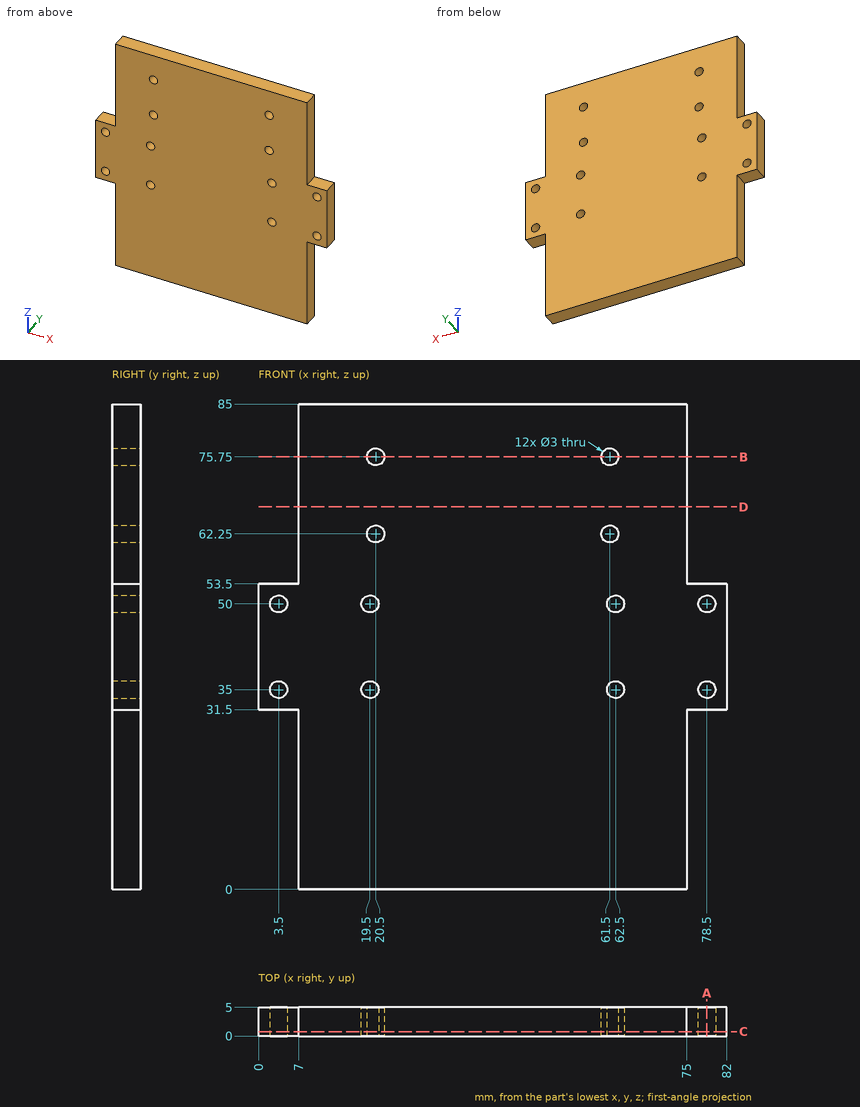
Print and shaded views of the part. All mm, measured from the part's lowest x, y and z. Round coordinates to 2 decimals unless told otherwise and drop trailing zeros. Order: outer loops, then holes, each group sorted by start corner. A loop starts at its lowest first (then second) coordinate and runs counter-clockwise, first axis right, second up.
Q1. Slice it at D-D (z = 67). Write the cut outline in (x, y), and give its area (3 significant figures).
Q2. Slice it at A-A (x = 78.5). Write the cut outline in (y, z), and give its area (3 significant figures).
Q3. Wall check: L1, parallel to X at y = 1.15, z = 76; L2, parallel to Z at x = 3, y = 2.9; L3, parallel to Z at x = 20.5, y = 1.7. Give the ranges that are in metal, low to high.
Q4. Drop flat-ended pins along their axis: pin 1 (5 mm diameter, centred on x = 62.5, z = 35, fed in from +Y); pin 2 (1.5 mm diameter, centred on y = 2, z = 23, fed in from +X); pin 3 (3 mm diameter, centred on y = 1.5, z = 71, fed in from -X); pin 4 (1.5 mm diameter, centred on x = 79, y = 1.5, fed in from +Z). Give the stop position or say it passes through.
Q5. Slice it at C-C (y = 0.75). State how many separate pieces and enclosed holes the cut face has, and give its area (3 significant figures).
Q6. Slice it at B-B (z = 75.75). Write the cut outline in (x, y), and give its area (3 significant figures).
Results below:
1. outline: (7, 0) - (75, 0) - (75, 5) - (7, 5) - close
1. area: 340 mm2
2. outline: (0, 31.5) - (5, 31.5) - (5, 33.5) - (0, 33.5) - close; (0, 36.5) - (5, 36.5) - (5, 48.5) - (0, 48.5) - close; (0, 51.5) - (5, 51.5) - (5, 53.5) - (0, 53.5) - close
2. area: 80.0 mm2
3. L1: x = 7 to 19.02, 21.98 to 60.02, 62.98 to 75
3. L2: z = 31.5 to 33.59, 36.41 to 48.59, 51.41 to 53.5
3. L3: z = 0 to 33.88, 36.12 to 48.88, 51.12 to 60.75, 63.75 to 74.25, 77.25 to 85
4. pin 1: stops at y = 5
4. pin 2: stops at x = 75
4. pin 3: stops at x = 7
4. pin 4: stops at z = 53.5
5. separate pieces: 1
5. enclosed holes: 12
5. area: 6,000 mm2
6. outline: (7, 0) - (19, 0) - (19, 5) - (7, 5) - close; (22, 0) - (60, 0) - (60, 5) - (22, 5) - close; (63, 0) - (75, 0) - (75, 5) - (63, 5) - close
6. area: 310 mm2
